The listing builds one solid part. Answer for the finished solid, in the listing's coordinates (mm). A direction names the side the tool comes from. Coordinates: 2 decimals unless noted, no trailing zeros. Loops run counter-clockwise (first coordinate to the right, second up) from the corner with the lowest first, then second, coordinate; pieces in that order, holes last. Notation, with made-up numbers: (46.5, 71.5) - (90.5, 71.5) arc R14 ccw to (90.5, 96.5) - close; hole circle Ø3 at (49.5, 70). An arc over 180 degrees is marked (long way). Put each result on its own line as item: value.
```python
from build123d import *

# Parameters (mm, degrees)
SKETCH1_W           = 70
SKETCH1_H           = 70
BOSS_EXTRUDE2_DEPTH = 7
CUT_EXTRUDE1_DEPTH  = 5
SKETCH9_W           = 70
SKETCH9_H           = 70
BOSS_EXTRUDE3_DEPTH = 5
CUT_EXTRUDE11_DEPTH = 100.242128151
SKETCH21_R          = 3
CUT_EXTRUDE12_DEPTH = 2
CUT_EXTRUDE13_START = -2
SKETCH22_W          = 70
SKETCH22_H          = 70
CUT_EXTRUDE13_DEPTH = 2
SKETCH27_R          = 3
CUT_EXTRUDE27_DEPTH = 2
SKETCH28_R          = 3
CUT_EXTRUDE28_DEPTH = 2
CUT_EXTRUDE29_DEPTH = 5
CUT_EXTRUDE30_DEPTH = 5
CHAMFER1_SIZE       = 1.5


with BuildPart() as part:
    # Sketch1 → Boss-Extrude2 (new body)
    with BuildSketch(Plane(origin=(0, 0, 0), x_dir=(1, 0, 0), z_dir=(0, 1, 0))):
        with Locations((35, 35)):
            Rectangle(SKETCH1_W, SKETCH1_H)
    extrude(amount=BOSS_EXTRUDE2_DEPTH)

    # Sketch3 → Cut-Extrude1 (cut)
    with BuildSketch(Plane(origin=(0, 7, 0), x_dir=(1, 0, 0), z_dir=(0, 1, 0))):
        with BuildLine():
            Line((2.5, 57.5), (2.5, 12.5))
            ThreePointArc((2.5, 12.5), (5.428932188, 5.428932188), (12.5, 2.5))
            Line((12.5, 2.5), (57.5, 2.5))
            ThreePointArc((57.5, 2.5), (64.571067812, 5.428932188), (67.5, 12.5))
            Line((67.5, 12.5), (67.5, 57.5))
            ThreePointArc((67.5, 57.5), (64.571067812, 64.571067812), (57.5, 67.5))
            Line((57.5, 67.5), (12.5, 67.5))
            ThreePointArc((12.5, 67.5), (5.428932188, 64.571067812), (2.5, 57.5))
        make_face()
    extrude(amount=-CUT_EXTRUDE1_DEPTH, mode=Mode.SUBTRACT)

    # Sketch9 → Boss-Extrude3 (add)
    with BuildSketch(Plane.XZ):
        with Locations((35, -35)):
            Rectangle(SKETCH9_W, SKETCH9_H)
    extrude(amount=BOSS_EXTRUDE3_DEPTH)

    # Sketch20 → Cut-Extrude11 (cut, through all)
    with BuildSketch(Plane(origin=(0, 2, 0), x_dir=(1, 0, 0), z_dir=(0, 1, 0))):
        with BuildLine():
            Line((13.745191882, 7.5), (56.254808118, 7.5))
            ThreePointArc((56.254808118, 7.5), (57.5, 12.5), (62.5, 13.745191882))
            Line((62.5, 13.745191882), (62.5, 56.254808118))
            ThreePointArc((62.5, 56.254808118), (57.5, 57.5), (56.254808118, 62.5))
            Line((56.254808118, 62.5), (13.745191882, 62.5))
            ThreePointArc((13.745191882, 62.5), (12.5, 57.5), (7.5, 56.254808118))
            Line((7.5, 56.254808118), (7.5, 13.745191882))
            ThreePointArc((7.5, 13.745191882), (12.5, 12.5), (13.745191882, 7.5))
        make_face()
    extrude(amount=-CUT_EXTRUDE11_DEPTH, mode=Mode.SUBTRACT)

    # Sketch21 → Cut-Extrude12 (cut)
    with BuildSketch(Plane(origin=(0, 2, 0), x_dir=(1, 0, 0), z_dir=(0, 1, 0))):
        with Locations(Location((8.964466094, 61.035533906, 0), (0, 0, 270))):
            Circle(SKETCH21_R)
        with Locations(Location((61.035533906, 61.035533906, 0), (0, 0, 270))):
            Circle(SKETCH21_R)
        with Locations(Location((61.035533906, 8.964466094, 0), (0, 0, 270))):
            Circle(SKETCH21_R)
        with Locations(Location((8.964466094, 8.964466094, 0), (0, 0, 270))):
            Circle(SKETCH21_R)
    extrude(amount=-CUT_EXTRUDE12_DEPTH, mode=Mode.SUBTRACT)

    # Sketch22 → Cut-Extrude13 (cut)
    with BuildSketch(Plane.XZ.offset(5).offset(CUT_EXTRUDE13_START)):
        with Locations((35, -35)):
            Rectangle(SKETCH22_W, SKETCH22_H)
        with BuildLine():
            Line((7.5, -13.745191882), (7.5, -56.254808118))
            ThreePointArc((7.5, -56.254808118), (12.5, -57.5), (13.745191882, -62.5))
            Line((13.745191882, -62.5), (56.254808118, -62.5))
            ThreePointArc((56.254808118, -62.5), (57.5, -57.5), (62.5, -56.254808118))
            Line((62.5, -56.254808118), (62.5, -13.745191882))
            ThreePointArc((62.5, -13.745191882), (57.5, -12.5), (56.254808118, -7.5))
            Line((56.254808118, -7.5), (13.745191882, -7.5))
            ThreePointArc((13.745191882, -7.5), (12.5, -12.5), (7.5, -13.745191882))
        make_face(mode=Mode.SUBTRACT)
    extrude(amount=CUT_EXTRUDE13_DEPTH, mode=Mode.SUBTRACT)

    # Sketch27 → Cut-Extrude27 (cut)
    with BuildSketch(Plane.ZY):
        with Locations((-62.5, 2)):
            Circle(SKETCH27_R)
        with Locations((-7.5, 2)):
            Circle(SKETCH27_R)
    extrude(amount=-CUT_EXTRUDE27_DEPTH, mode=Mode.SUBTRACT)

    # Sketch28 → Cut-Extrude28 (cut)
    with BuildSketch(Plane.XY):
        with Locations((7.5, 2)):
            Circle(SKETCH28_R)
        with Locations((62.5, 2)):
            Circle(SKETCH28_R)
    extrude(amount=-CUT_EXTRUDE28_DEPTH, mode=Mode.SUBTRACT)

    # Mirror2: part across plane


with BuildPart() as part_1:
    add(part.part)
    add(part.part.mirror(Plane(origin=(0, 7, -70), x_dir=(1, 0, 0), z_dir=(0, 0, 1))))

    # Mirror3: part across plane


with BuildPart() as part_2:
    add(part_1.part)
    add(part_1.part.mirror(Plane(origin=(70, 7, 0), x_dir=(0, 0, 1), z_dir=(-1, 0, 0))))

    # Sketch30 → Cut-Extrude29 (cut)
    with BuildSketch(Plane(origin=(0, 7, 0), x_dir=(1, 0, 0), z_dir=(0, 1, 0))):
        with BuildLine():
            Line((2, 57.5), (2, 12.5))
            ThreePointArc((2, 12.5), (5.075378798, 5.075378798), (12.5, 2))
            Line((12.5, 2), (57.5, 2))
            ThreePointArc((57.5, 2), (64.924621202, 5.075378798), (68, 12.5))
            Line((68, 12.5), (68, 57.5))
            ThreePointArc((68, 57.5), (64.924621202, 64.924621202), (57.5, 68))
            Line((57.5, 68), (12.5, 68))
            ThreePointArc((12.5, 68), (5.075378798, 64.924621202), (2, 57.5))
        make_face()
    extrude(amount=-CUT_EXTRUDE29_DEPTH, mode=Mode.SUBTRACT)

    # Sketch31 → Cut-Extrude30 (cut)
    with BuildSketch(Plane(origin=(0, 7, 0), x_dir=(1, 0, 0), z_dir=(0, 1, 0))):
        with BuildLine():
            Line((68, 82.5), (68, 127.5))
            ThreePointArc((68, 127.5), (64.924621202, 134.924621202), (57.5, 138))
            Line((57.5, 138), (12.5, 138))
            ThreePointArc((12.5, 138), (5.075378798, 134.924621202), (2, 127.5))
            Line((2, 127.5), (2, 82.5))
            ThreePointArc((2, 82.5), (5.075378798, 75.075378798), (12.5, 72))
            Line((12.5, 72), (57.5, 72))
            ThreePointArc((57.5, 72), (64.924621202, 75.075378798), (68, 82.5))
        make_face()
        with BuildLine():
            Line((82.5, 72), (127.5, 72))
            ThreePointArc((127.5, 72), (134.924621202, 75.075378798), (138, 82.5))
            Line((138, 82.5), (138, 127.5))
            ThreePointArc((138, 127.5), (134.924621202, 134.924621202), (127.5, 138))
            Line((127.5, 138), (82.5, 138))
            ThreePointArc((82.5, 138), (75.075378798, 134.924621202), (72, 127.5))
            Line((72, 127.5), (72, 82.5))
            ThreePointArc((72, 82.5), (75.075378798, 75.075378798), (82.5, 72))
        make_face()
        with BuildLine():
            Line((72, 57.5), (72, 12.5))
            ThreePointArc((72, 12.5), (75.075378798, 5.075378798), (82.5, 2))
            Line((82.5, 2), (127.5, 2))
            ThreePointArc((127.5, 2), (134.924621202, 5.075378798), (138, 12.5))
            Line((138, 12.5), (138, 57.5))
            ThreePointArc((138, 57.5), (134.924621202, 64.924621202), (127.5, 68))
            Line((127.5, 68), (82.5, 68))
            ThreePointArc((82.5, 68), (75.075378798, 64.924621202), (72, 57.5))
        make_face()
    extrude(amount=-CUT_EXTRUDE30_DEPTH, mode=Mode.SUBTRACT)

    # Chamfer1
    chamfer1_edges = [part_2.edges().sort_by_distance(p)[0] for p in [
        (5.075378798, 7, -64.924621202),
        (2, 7, -35),
        (5.075378798, 7, -5.075378798),
        (35, 7, -2),
        (64.924621202, 7, -5.075378798),
        (68, 7, -35),
        (64.924621202, 7, -64.924621202),
        (35, 7, -68),
        (64.924621202, 7, -134.924621202),
        (35, 7, -138),
        (5.075378798, 7, -134.924621202),
        (2, 7, -105),
        (5.075378798, 7, -75.075378798),
        (35, 7, -72),
        (64.924621202, 7, -75.075378798),
        (68, 7, -105),
        (75.075378798, 7, -5.075378798),
        (105, 7, -2),
        (134.924621202, 7, -5.075378798),
        (138, 7, -35),
        (134.924621202, 7, -64.924621202),
        (105, 7, -68),
        (75.075378798, 7, -64.924621202),
        (72, 7, -35),
        (75.075378798, 7, -75.075378798),
        (105, 7, -72),
        (134.924621202, 7, -75.075378798),
        (138, 7, -105),
        (134.924621202, 7, -134.924621202),
        (105, 7, -138),
        (75.075378798, 7, -134.924621202),
        (72, 7, -105),
    ]]
    chamfer(chamfer1_edges, length=CHAMFER1_SIZE)


solid = part_2.part
```
1) Straight lines are drawn through the part: L1, parallel to X at y = 1.25, z = -100; L2, parallel to X at y = 2.75, z = -46; L3, parallel to Z at x = 26, y = 5.5. For each, find the intervals that lie inside material, in ascending order. Write a range as [from, to].
Found:
L1: x = [0, 7.5], [62.5, 77.5], [132.5, 140]
L2: x = [0, 2], [68, 72], [138, 140]
L3: z = [-140, -138], [-72, -68], [-2, 0]
2) The part is cut by section A-A (x = 117.5). Give the vertices of the cut face in (y, z).
Found:
outline: (-3, -140) - (7, -140) - (7, -139.5) - (5.5, -138) - (2, -138) - (2, -132.5) - (-3, -132.5) - close; (-3, -77.5) - (2, -77.5) - (2, -72) - (5.5, -72) - (7, -70.5) - (7, -69.5) - (5.5, -68) - (2, -68) - (2, -62.5) - (-3, -62.5) - close; (-3, -7.5) - (2, -7.5) - (2, -2) - (5.5, -2) - (7, -0.5) - (7, 0) - (-3, 0) - close
3) For a pull along Y with two mould halves and no side action, classify faces 4 (the face through (2, 2, -132)), 5 (the face through (79, 0, -131)), 6 (the face through (134.84, 3.77, -74.99)) as pulls with the +Y half, pulls with the -Y half, needs draft (parallel to the pull), parting line crosses it, or undercut.
Found:
face 4: undercut
face 5: pulls with the +Y half
face 6: needs draft
4) Each of these flat-tipped pins is pushed along its axis until it touches: pin 1 (5 mm diameter, centred on x = 8, z = -131.5, fed in from +Y); pin 2 (1.8 mm diameter, centred on x = 131, z = -9, fed in from +Y); pin 3 (3.5 mm diameter, centred on y = 2, z = -132.5, fed in from -X); pin 4 (4 mm diameter, centred on x = 115, y = -0.5, fed in from +Z). Where does it stop, or does it pass through?
Found:
pin 1: stops at y = 2
pin 2: stops at y = 0
pin 3: stops at x = 2
pin 4: stops at z = 0
5) For faces 1 (the face through (7.5, 0, -105)), 2 (the face through (131, 0, -61)), 3 (the face through (59.5, 2.1, -139)), determine the directions among +Z, -Z, +X, -X, +Y, -Y from which every point of the face is accessible in a straight line to the end or side of a thin tool.
Found:
face 1: +Y, -Y
face 2: +Y
face 3: -Z
6) The part is cut by section B-B (z = -123). Give the vertices of the cut face in (x, y).
Found:
outline: (0, -3) - (7.5, -3) - (7.5, 2) - (2, 2) - (2, 5.5) - (0.5, 7) - (0, 7) - close; (62.5, -3) - (77.5, -3) - (77.5, 2) - (72, 2) - (72, 5.5) - (70.5, 7) - (69.5, 7) - (68, 5.5) - (68, 2) - (62.5, 2) - close; (132.5, -3) - (140, -3) - (140, 7) - (139.5, 7) - (138, 5.5) - (138, 2) - (132.5, 2) - close
